```python
from build123d import *

# Parameters (mm, degrees)
BOSS_EXTRUDE1_DEPTH = 1.25
BOSS_EXTRUDE5_DEPTH = 2.5
SKETCH6_W           = 5
SKETCH6_H           = 4
CUT_EXTRUDE1_DEPTH  = 1.25
CUT_EXTRUDE2_DEPTH  = 2.5


with BuildPart() as part:
    # Sketch2 → Boss-Extrude1 (new body, symmetric)
    with BuildSketch(Plane(origin=(0, 0, 0), x_dir=(1, 0, 0), z_dir=(0, 1, 0))):
        with BuildLine():
            Line((-16.109808132, 47.688266684), (-8.537351427, 75.949059844))
            ThreePointArc((-8.537351427, 75.949059844), (0, 82.5), (8.537351427, 75.949059844))
            Line((8.537351427, 75.949059844), (16.109808132, 47.688266684))
            ThreePointArc((16.109808132, 47.688266684), (18.609958913, 43.946526618), (22.871288916, 42.5))
            Line((22.871288916, 42.5), (50, 42.5))
            ThreePointArc((50, 42.5), (60.606601718, 38.106601718), (65, 27.5))
            Line((65, 27.5), (65, -27.5))
            ThreePointArc((65, -27.5), (53.284271247, -55.784271247), (25, -67.5))
            Line((25, -67.5), (-25, -67.5))
            ThreePointArc((-25, -67.5), (-53.284271247, -55.784271247), (-65, -27.5))
            Line((-65, -27.5), (-65, 27.5))
            ThreePointArc((-65, 27.5), (-60.606601718, 38.106601718), (-50, 42.5))
            Line((-50, 42.5), (-22.871288916, 42.5))
            ThreePointArc((-22.871288916, 42.5), (-18.609958913, 43.946526618), (-16.109808132, 47.688266684))
        make_face()
        with BuildLine():
            Line((6.122536861, 75.302012231), (13.694993566, 47.041219072))
            ThreePointArc((13.694993566, 47.041219072), (17.08805534, 41.963143267), (22.871288916, 40))
            Line((22.871288916, 40), (50, 40))
            ThreePointArc((50, 40), (58.838834765, 36.338834765), (62.5, 27.5))
            Line((62.5, 27.5), (62.5, -27.5))
            ThreePointArc((62.5, -27.5), (51.516504294, -54.016504294), (25, -65))
            Line((25, -65), (-25, -65))
            ThreePointArc((-25, -65), (-51.516504294, -54.016504294), (-62.5, -27.5))
            Line((-62.5, -27.5), (-62.5, 27.5))
            ThreePointArc((-62.5, 27.5), (-58.838834765, 36.338834765), (-50, 40))
            Line((-50, 40), (-22.871288916, 40))
            ThreePointArc((-22.871288916, 40), (-17.08805534, 41.963143267), (-13.694993566, 47.041219072))
            Line((-13.694993566, 47.041219072), (-6.122536861, 75.302012231))
            ThreePointArc((-6.122536861, 75.302012231), (0, 80), (6.122536861, 75.302012231))
        make_face(mode=Mode.SUBTRACT)
    extrude(amount=BOSS_EXTRUDE1_DEPTH, both=True)

    # Sketch5 → Boss-Extrude5 (add)
    with BuildSketch(Plane(origin=(0, 1.25, 0), x_dir=(1, 0, 0), z_dir=(0, 1, 0))):
        with BuildLine():
            ThreePointArc((-62.5, 27.5), (-53.661165235, 31.161165235), (-50, 40))
            ThreePointArc((-50, 40), (-58.838834765, 36.338834765), (-62.5, 27.5))
        make_face()
        with BuildLine():
            ThreePointArc((50, 40), (53.661165235, 31.161165235), (62.5, 27.5))
            ThreePointArc((62.5, 27.5), (58.838834765, 36.338834765), (50, 40))
        make_face()
        with BuildLine():
            ThreePointArc((-62.5, -27.5), (-54.791585286, -34.595919329), (-58.473512014, -44.404851181))
            ThreePointArc((-58.473512014, -44.404851181), (-61.479492188, -36.188880811), (-62.5, -27.5))
        make_face()
        with BuildLine():
            ThreePointArc((62.5, -27.5), (54.791585286, -34.595919329), (58.473512014, -44.404851181))
            ThreePointArc((58.473512014, -44.404851181), (61.479492187, -36.188880811), (62.5, -27.5))
        make_face()
    extrude(amount=-BOSS_EXTRUDE5_DEPTH)

    # Sketch6 → Cut-Extrude1 (cut)
    with BuildSketch(Plane(origin=(0, 1.25, 0), x_dir=(1, 0, 0), z_dir=(0, 1, 0))):
        with Locations((0, 81.25)):
            Rectangle(SKETCH6_W, SKETCH6_H)
        with BuildLine():
            Line((-20.493193447, 42.916333701), (-19.643873637, 40.565024308))
            ThreePointArc((-19.643873637, 40.565024308), (-17.08805534, 41.963143267), (-15.076081678, 44.070014354))
            Line((-15.076081678, 44.070014354), (-17.127452004, 45.498957945))
            ThreePointArc((-17.127452004, 45.498957945), (-18.609958913, 43.946526618), (-20.493193447, 42.916333701))
        make_face()
        with BuildLine():
            Line((20.493193447, 42.916333701), (19.643873637, 40.565024308))
            ThreePointArc((19.643873637, 40.565024308), (17.08805534, 41.963143267), (15.076081678, 44.070014354))
            Line((15.076081678, 44.070014354), (17.127452004, 45.498957945))
            ThreePointArc((17.127452004, 45.498957945), (18.609958913, 43.946526618), (20.493193447, 42.916333701))
        make_face()
        with BuildLine():
            Line((-53.284271247, -55.784271247), (-51.516504294, -54.016504294))
            ThreePointArc((-51.516504294, -54.016504294), (-49.689746158, -55.725280064), (-47.753133619, -57.308470449))
            Line((-47.753133619, -57.308470449), (-49.270009194, -59.295701812))
            ThreePointArc((-49.270009194, -59.295701812), (-51.335729235, -57.606965401), (-53.284271247, -55.784271247))
        make_face()
        with BuildLine():
            Line((49.270009194, -59.295701812), (47.753133619, -57.308470449))
            ThreePointArc((47.753133619, -57.308470449), (49.689746158, -55.725280064), (51.516504294, -54.016504294))
            Line((51.516504294, -54.016504294), (53.284271247, -55.784271247))
            ThreePointArc((53.284271247, -55.784271247), (51.335729235, -57.606965401), (49.270009194, -59.295701812))
        make_face()
        with Locations((0, -66.5)):
            Rectangle(SKETCH6_W, SKETCH6_H)
    extrude(amount=-CUT_EXTRUDE1_DEPTH, mode=Mode.SUBTRACT)

    # Sketch7 → Cut-Extrude2 (cut)
    with BuildSketch(Plane(origin=(0, 1.25, 0), x_dir=(1, 0, 0), z_dir=(0, 1, 0))):
        with BuildLine():
            ThreePointArc((-62.5, 29.791666667), (-55.281618275, 32.781618275), (-52.291666667, 40))
            ThreePointArc((-52.291666667, 40), (-58.986148678, 36.486148678), (-62.5, 29.791666667))
        make_face()
        with BuildLine():
            ThreePointArc((52.291666667, 40), (58.986148678, 36.486148678), (62.5, 29.791666667))
            ThreePointArc((62.5, 29.791666667), (55.281618275, 32.781618275), (52.291666667, 40))
        make_face()
        with BuildLine():
            ThreePointArc((-59.600502093, -42.173283714), (-57.223551432, -35.175178049), (-62.5, -30))
            ThreePointArc((-62.5, -30), (-61.479492188, -36.188880811), (-59.600502093, -42.173283714))
        make_face()
        with BuildLine():
            ThreePointArc((62.5, -30), (61.479492187, -36.188880811), (59.600502093, -42.173283714))
            ThreePointArc((59.600502093, -42.173283714), (57.223551432, -35.175178049), (62.5, -30))
        make_face()
    extrude(amount=-CUT_EXTRUDE2_DEPTH, mode=Mode.SUBTRACT)


solid = part.part
```
Design review of the part built by this model. Coordinates are the model's own, in mm. A direction names the side the tool comes from. Give positions to 0.01 mm unless a question says otherwise; leave off trailing zeros. Order: outer loops, then holes, each group sorted by start corner. A loop starts at its lowest first (then second) coordinate and runs counter-clockwise, first axis right, second up. Notation, with made-up numbers: (1, 85.5) - (60, 85.5) arc R24 cw to (60, 112.5) - close; hole circle Ø11 at (-19.75, 27.25). An arc over 180 degrees is marked (long way). Use a Markdown table: item, result. Add a question column.
(1) Add section B-B on x = -40.5. Give the boundary of the cut face in (y, z), then the cut area to 3 significant figures.
(2) Add section A-A on z = 10. Give the boundary of the cut face in (x, y).
(3) Add section D-D on z = 33. Give the boundary of the cut face in (x, y).
(4) Add section C-C on y = 0.7. Give the number of separate pieces and of enclosed holes in the cut face, then the cut area to 3 significant figures.
(5) Mouldability with a two-part tool opening along Z and no side actions: class faces 1 (the face through (58.91, 0.02, -36.56)), 2 (the face through (-52.972, -0.26, 56.094)), 3 (the face through (64, 1.25, -5)), 4 (the face through (12.27, 0.02, -62.02)) as +Z half, -Z half, draft (parallel to the pull), parting line (faces both ways), or undercut.
(6) Clearance check with flat-ended pins moving along their axes: P1, Ø1.2, axis at x = 1, z = 66, coming from the +Y side; P2, Ø1.2, axis at x = -34, y = 0, coming from the +Z side; P3, Ø0.8, axis at x = 5.5, y = 0, coming from the -Z side. State where each tip first meets the part, or that it passes through.
(7) Wall thickness on probe 1 along X at (y, z) = (-1, 15); probe 2 along X at (y, z) = (0.4, -28.5); probe 3 along Z at (x, y) = (-57, -0.9): over which ranges is each line inside the solid? List them lowest first. Write a range as [from, to].
(8) Machinability: for faces 5 (the face through (-18, 0, -43)), 6 (the face through (53.565, 0.018, -31.259)), 7 (the face through (60.49, 0.02, -38.22)), which of the approach directions +Z, -Z, +X, -X, +Y, -Y give a long, thin tool a straight path to every point of the face, cutting with its end or side? Answer none if there is none.
Report:
| question | item | result |
|---|---|---|
| 1 | outline | (-1.25, -42.5) - (1.25, -42.5) - (1.25, -40) - (-1.25, -40) - close; (-1.25, 61.65) - (1.25, 61.65) - (1.25, 64.37) - (-1.25, 64.37) - close |
| 1 | area | 13.1 mm² |
| 2 | outline | (-65, -1.25) - (-62.5, -1.25) - (-62.5, 1.25) - (-65, 1.25) - close; (62.5, -1.25) - (65, -1.25) - (65, 1.25) - (62.5, 1.25) - close |
| 3 | outline | (-64.62, -1.25) - (-62.12, -1.25) - (-62.12, 1.25) - (-64.62, 1.25) - close; (-58.16, -1.25) - (-55.33, -1.25) - (-55.33, 1.25) - (-58.16, 1.25) - close; (55.33, -1.25) - (58.16, -1.25) - (58.16, 1.25) - (55.33, 1.25) - close; (62.12, -1.25) - (64.62, -1.25) - (64.62, 1.25) - (62.12, 1.25) - close |
| 4 | separate pieces | 6 |
| 4 | enclosed holes | 4 |
| 4 | area | 1,290 mm² |
| 5 | face 1 | undercut |
| 5 | face 2 | +Z half |
| 5 | face 3 | draft |
| 5 | face 4 | -Z half |
| 6 | P1 | stops at y = 0 |
| 6 | P2 | stops at z = 66.61 |
| 6 | P3 | stops at z = -80.88 |
| 7 | probe 1 | x = [-65, -62.5], [62.5, 65] |
| 7 | probe 2 | x = [-64.97, -57.6], [57.6, 64.97] |
| 7 | probe 3 | z = [-40.77, -38.11], [-31.4, -28.78], [30.43, 43.1], [47.05, 51.5] |
| 8 | face 5 | +Y |
| 8 | face 6 | +Y, -Y |
| 8 | face 7 | -Z, +X, +Y, -Y |
